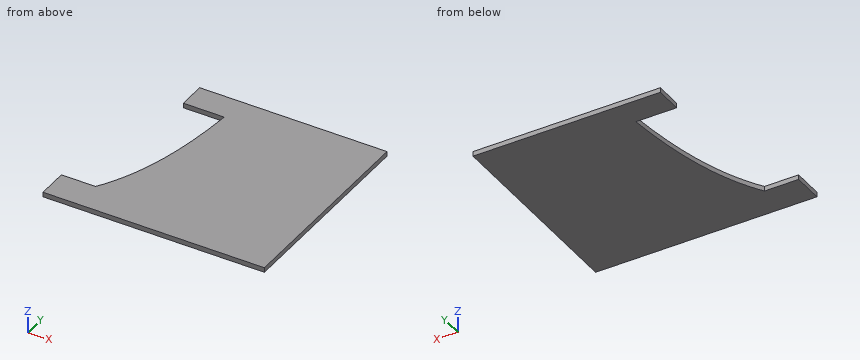
```python
from build123d import *

# Parameters (mm, degrees)
PAD_DEPTH = 14


with BuildPart() as part:
    # Sketch → Pad (new body)
    with BuildSketch(Plane.XY):
        with BuildLine():
            Line((0, 0), (650, 0))
            Line((650, 0), (650, 600))
            Line((650, 600), (100, 600))
            Line((100, 600), (100, 520))
            Line((100, 520), (220, 520))
            add(Edge.make_bspline(
                [(220, 520), (198.506592, 233.641052), (100, 90)],
                knots=[0, 0, 0, 1, 1, 1], degree=2))
            Line((100, 90), (0, 90))
            Line((0, 90), (0, 0))
        make_face()
    extrude(amount=PAD_DEPTH)


solid = part.part
```
Design review of the part built by this model. Coordinates are the model's own, in mm. Round coordinates to 2 decimals unless told otherwise and drop trailing zeros. Order: outer loops, then holes, each group sorted by start corner. A loop starts at its lowest first (then second) coordinate and runs counter-clockwise, first axis right, second up. Notation, with made-up numbers: (17.25, -12.75) - (67.25, -12.75) arc R11 ccw to (67.25, 1.25) - close; hole circle Ø8 at (55, 20.5). An arc over 180 degrees is marked (long way). One line per question, with ' | ' between items.
Item 1: Wall thickness on line 1 (X direction, y = 559.5, z = 10.25); line 2 (X direction, y = 396, z = 10.5): over which ranges is each line inside the solid? List them lowest first. Write a range as [from, to].
Checks:
line 1: [100, 650] | line 2: [206.07, 650]
Item 2: Take a section at A-A, the plane y = 529. Write out the cut boundary in (x, z), then the cut area to 3 significant figures.
Checks:
outline: (100, 0) - (650, 0) - (650, 14) - (100, 14) - close | area: 7,700 mm²
Item 3: For P1, Ø4, axis at y = 575, z = 9.5, coming from the -X side; P2, Ø8, axis at y = 267.5, z = 2.5, coming from the -X side, all flat-tipped, find the tip position at first contact; note any pin that passes through.
Checks:
P1: x = 100 | P2: x = 177.61
